from build123d import *

# Parameters (mm, degrees)
F0_W      = 70
F0_H      = 80
F1_DEPTH  = 3
F3_D      = 3
F7_DEPTH  = 3
F9_D      = 3
F11_D     = 3
F12_DEPTH = 25
F15_D     = 3
F17_D     = 3


with BuildPart() as f1:
    # F0 (on Top) → F1 (new body)
    with BuildSketch(Plane.XY):
        with Locations((35, 40)):
            Rectangle(F0_W, F0_H)
    extrude(amount=F1_DEPTH)

    # F3 (through all)
    with Locations(Plane.XY.offset(3)):
        with Locations((45, 61), (45, 37)):
            Hole(F3_D / 2)

    # F6 (on face) → F7 (join)
    with BuildSketch(Plane.XY.offset(3)):
        Polygon((35, -114.782403), (70, 0), (0, 0), (0, -114.782403), align=None)
    extrude(amount=-F7_DEPTH)

    # F9 (through all)
    with Locations(Plane.XY.offset(3)):
        with Locations((-41.79904, -36.838889), (43.20096, -36.838889)):
            Hole(F9_D / 2)

    # F11 (through all)
    with Locations(Plane.XY.offset(3)):
        with Locations((-13.970835, -106.033295), (5.029165, -106.033295)):
            Hole(F11_D / 2)

    # F5 (on face) → F12 (cut)
    with BuildSketch(Plane.XY.offset(3)):
        with BuildLine():
            ThreePointArc((62.5, 75), (60, 77.5), (57.5, 75))
            Line((57.5, 75), (57.5, 25))
            ThreePointArc((57.5, 25), (60, 22.5), (62.5, 25))
            Line((62.5, 25), (62.5, 75))
        make_face()
    extrude(amount=-F12_DEPTH, mode=Mode.SUBTRACT)

    # F14: F1 across plane


with BuildPart() as f1_1:
    add(f1.part)
    add(f1.part.mirror(Plane.YZ))

    # F15 (through all)
    with Locations(Plane.XY.offset(3)):
        with Locations((29.87123, -73.830966)):
            Hole(F15_D / 2)

    # F17 (through all)
    with Locations(Plane.XY.offset(3)):
        with Locations((-44.679251, 0)):
            Hole(F17_D / 2)


solid = f1_1.part
Design review of the part built by this model. Coordinates are the model's own, in mm. Round coordinates to 2 decimals unless told otherwise and drop trailing zeros. Write each loop counter-clockwise with the first axis right and the second up, starting at its lowest first coordinate (ties: lowest second). Pieces come first, ordered by that corner, then holes. Notation, with made-up numbers: (79, 71) - (136, 71) arc R24 ccw to (136, 95) - close; hole circle Ø11 at (-22.5, 70). An arc over 180 degrees is marked (long way). Return JSON: item names as keys, results as strings. Group by question number.
Item 1: We need section A-A on y = 56.5. Write out the cut boundary in (x, z), and give its area (3 significant figures).
Item 2: We need section B-B on x = -59.5. Write out the cut boundary in (y, z), and give its area (3 significant figures).
Item 3: Insertion check: P1, Ø3.5, axis at x = 45, y = 61, coming from the -Z side; P2, Ø1, axis at y = -15.5, z = 1.5, coming from the +X side. Each pin has a flat end and moves straight along its axis. Give the tip position at first contact, or say it passes through.
Item 4: We need section D-D on x = 60. Write out the cut boundary in (y, z), and give its area (3 significant figures).
Item 5: For probe 1 along X at (y, z) = (70, 0.35); probe 2 along X at (y, z) = (-0.5, 0.85); probe 3 along X at (y, z) = (-19.5, 0.6), list the stretches that pass through material, from the lowest coordinate up. Write a range as [from, to].
Item 6: We need section C-C on z = 0.7. Give the number of separate pieces and of enclosed holes in the cut face, and give its area (3 significant figures).
Model answer:
{
 "1": {"outline": "(-70, 0) - (-62.5, 0) - (-62.5, 3) - (-70, 3) - close; (-57.5, 0) - (57.5, 0) - (57.5, 3) - (-57.5, 3) - close; (62.5, 0) - (70, 0) - (70, 3) - (62.5, 3) - close", "area": "390 mm²"},
 "2": {"outline": "(-34.43, 0) - (22.55, 0) - (22.55, 3) - (-34.43, 3) - close; (77.45, 0) - (80, 0) - (80, 3) - (77.45, 3) - close", "area": "179 mm²"},
 "3": {"P1": "stops at z = 0", "P2": "stops at x = 65.43"},
 "4": {"outline": "(-32.79, 0) - (22.5, 0) - (22.5, 3) - (-32.79, 3) - close; (77.5, 0) - (80, 0) - (80, 3) - (77.5, 3) - close", "area": "173 mm²"},
 "5": {"probe 1": "x = [-70, -62.5], [-57.5, 57.5], [62.5, 70]", "probe 2": "x = [-69.85, -46.09], [-43.27, 69.85]", "probe 3": "x = [-64.05, 64.05]"},
 "6": {"separate pieces": "1", "enclosed holes": "12", "area": "22,600 mm²"}
}
